Autodesk Inventor part; units mm, degrees
ref_plane "YZ Plane" through (0, 0, 0) normal (1, 0, 0) x (0, 1, 0)
ref_plane "XZ Plane" through (0, 0, 0) normal (0, 1, 0) x (-1, 0, 0)
ref_plane "XY Plane" through (0, 0, 0) normal (0, 0, 1) x (1, 0, 0)
sketch "Sketch1" plane through (0, 0, 0) normal (0, 1, 0) x (-1, 0, 0)
  line L0 (-62, 109.5) -> (62, 109.5)
  line L1 (62, 109.5) -> (62, -109.5)
  line L2 (62, -109.5) -> (-62, -109.5)
  line L3 (-62, -109.5) -> (-62, 109.5)
  line L4 (-62, 109.5) -> (62, -109.5) construction
  line L5 (62, 109.5) -> (-62, -109.5) construction
  point P0 (0, 0)
  dimension "d0" = 219
  dimension "d1" = 124
extrude "Extrusion1" add sketch "Sketch1" along normal blind 0.1
chamfer "Chamfer1" distance 4 angle 45 1 edges at (-62, 0.05, 109.5)
sketch "Sketch2" plane through (0, 0.1, 0) normal (0, 1, 0) x (1, 0, 0)
  line L0 (-35.5, -100.5) -> (-35.5, -70.5)
  line L1 (-35.5, -70.5) -> (-57.5, -70.5)
  line L2 (-62, 109.5) -> (-62, -109.5)
  line L3 (-62, -109.5) -> (62, -109.5)
  arc A0 (-57.5, -99) -> (-56, -100.5) centre (-57.5, -100.5) ccw
  line L4 (-35.5, -100.5) -> (-56, -100.5)
  line L5 (-57.5, -99) -> (-57.5, -70.5)
  line L6 (62, -109.5) -> (62, 109.5)
  line L7 (-35.5, -43.5) -> (-35.5, -13.5)
  line L8 (-35.5, -43.5) -> (-56, -43.5)
  line L9 (-35.5, -13.5) -> (-57.5, -13.5)
  line L10 (-57.5, -42) -> (-57.5, -13.5)
  arc A1 (-57.5, -42) -> (-56, -43.5) centre (-57.5, -43.5) ccw
  line L11 (-35.5, 13.5) -> (-35.5, 43.5)
  line L12 (-35.5, 13.5) -> (-56, 13.5)
  line L13 (-35.5, 43.5) -> (-57.5, 43.5)
  line L14 (-57.5, 15) -> (-57.5, 43.5)
  arc A2 (-57.5, 15) -> (-56, 13.5) centre (-57.5, 13.5) ccw
  line L15 (-35.5, 70.5) -> (-35.5, 100.5)
  line L16 (-35.5, 70.5) -> (-56, 70.5)
  line L17 (-35.5, 100.5) -> (-57.5, 100.5)
  line L18 (-57.5, 72) -> (-57.5, 100.5)
  arc A3 (-57.5, 72) -> (-56, 70.5) centre (-57.5, 70.5) ccw
  line L19 (-4.5, -100.5) -> (-4.5, -70.5)
  line L20 (-4.5, -100.5) -> (-25, -100.5)
  line L21 (-4.5, -70.5) -> (-26.5, -70.5)
  line L22 (-26.5, -99) -> (-26.5, -70.5)
  arc A4 (-26.5, -99) -> (-25, -100.5) centre (-26.5, -100.5) ccw
  line L23 (-4.5, -43.5) -> (-4.5, -13.5)
  line L24 (-4.5, -43.5) -> (-25, -43.5)
  line L25 (-4.5, -13.5) -> (-26.5, -13.5)
  line L26 (-26.5, -42) -> (-26.5, -13.5)
  arc A5 (-26.5, -42) -> (-25, -43.5) centre (-26.5, -43.5) ccw
  line L27 (-4.5, 13.5) -> (-4.5, 43.5)
  line L28 (-4.5, 13.5) -> (-25, 13.5)
  line L29 (-4.5, 43.5) -> (-26.5, 43.5)
  line L30 (-26.5, 15) -> (-26.5, 43.5)
  arc A6 (-26.5, 15) -> (-25, 13.5) centre (-26.5, 13.5) ccw
  line L31 (-4.5, 70.5) -> (-4.5, 100.5)
  line L32 (-4.5, 70.5) -> (-25, 70.5)
  line L33 (-4.5, 100.5) -> (-26.5, 100.5)
  line L34 (-26.5, 72) -> (-26.5, 100.5)
  arc A7 (-26.5, 72) -> (-25, 70.5) centre (-26.5, 70.5) ccw
  line L35 (26.5, -100.5) -> (26.5, -70.5)
  line L36 (26.5, -100.5) -> (6, -100.5)
  line L37 (26.5, -70.5) -> (4.5, -70.5)
  line L38 (4.5, -99) -> (4.5, -70.5)
  arc A8 (4.5, -99) -> (6, -100.5) centre (4.5, -100.5) ccw
  line L39 (26.5, -43.5) -> (26.5, -13.5)
  line L40 (26.5, -43.5) -> (6, -43.5)
  line L41 (26.5, -13.5) -> (4.5, -13.5)
  line L42 (4.5, -42) -> (4.5, -13.5)
  arc A9 (4.5, -42) -> (6, -43.5) centre (4.5, -43.5) ccw
  line L43 (26.5, 13.5) -> (26.5, 43.5)
  line L44 (26.5, 13.5) -> (6, 13.5)
  line L45 (26.5, 43.5) -> (4.5, 43.5)
  line L46 (4.5, 15) -> (4.5, 43.5)
  arc A10 (4.5, 15) -> (6, 13.5) centre (4.5, 13.5) ccw
  line L47 (26.5, 70.5) -> (26.5, 100.5)
  line L48 (26.5, 70.5) -> (6, 70.5)
  line L49 (26.5, 100.5) -> (4.5, 100.5)
  line L50 (4.5, 72) -> (4.5, 100.5)
  arc A11 (4.5, 72) -> (6, 70.5) centre (4.5, 70.5) ccw
  line L51 (57.5, -100.5) -> (57.5, -70.5)
  line L52 (57.5, -100.5) -> (37, -100.5)
  line L53 (57.5, -70.5) -> (35.5, -70.5)
  line L54 (35.5, -99) -> (35.5, -70.5)
  arc A12 (35.5, -99) -> (37, -100.5) centre (35.5, -100.5) ccw
  line L55 (57.5, -43.5) -> (57.5, -13.5)
  line L56 (57.5, -43.5) -> (37, -43.5)
  line L57 (57.5, -13.5) -> (35.5, -13.5)
  line L58 (35.5, -42) -> (35.5, -13.5)
  arc A13 (35.5, -42) -> (37, -43.5) centre (35.5, -43.5) ccw
  line L59 (57.5, 13.5) -> (57.5, 43.5)
  line L60 (57.5, 13.5) -> (37, 13.5)
  line L61 (57.5, 43.5) -> (35.5, 43.5)
  line L62 (35.5, 15) -> (35.5, 43.5)
  arc A14 (35.5, 15) -> (37, 13.5) centre (35.5, 13.5) ccw
  line L63 (57.5, 70.5) -> (57.5, 100.5)
  line L64 (57.5, 70.5) -> (37, 70.5)
  line L65 (57.5, 100.5) -> (35.5, 100.5)
  line L66 (35.5, 72) -> (35.5, 100.5)
  arc A15 (35.5, 72) -> (37, 70.5) centre (35.5, 70.5) ccw
  dimension "d46" = 1.5
  dimension "d47" = 30
  dimension "d50" = 9
  dimension "d51" = 4.5
  dimension "d62" = 57
  dimension "d65" = 31
  dimension "d77" = 22
extrude "Extrusion2" cut sketch "Sketch2" against normal through all
fillet "Fillet1" radius 1 5 edges at (62, 0.05, 109.5) (-58, 0.05, 109.5) (-62, 0.05, 105.5) (62, 0.05, -109.5) (-62, 0.05, -109.5)
sketch "Sketch3" plane through (0, 0.1, 0) normal (0, 1, 0) x (1, 0, 0)
  line L0 (-62, 108.5) -> (-62, -105.0858)
  line L1 (62, -108.5) -> (62, 108.5)
  line L2 (-57.5858, -109.5) -> (61, -109.5)
  line L3 (61, 109.5) -> (-61, 109.5)
  point P0 (0, 0)
  point P1 (-47, -105.5)
  point P2 (47, -105.5)
  point P3 (47, 105.5)
  point P4 (-47, 105.5)
  point P5 (-47, 0)
  point P6 (47, 0)
  dimension "d90" = 15
  dimension "d91" = 15
  dimension "d92" = 4
  dimension "d93" = 4
hole "Hole1" at (-47, 0.1, 105.5) at (47, 0.1, 105.5) at (47, 0.1, -105.5) at (-47, 0.1, -105.5) at (-47, 0.1, 0) at (47, 0.1, 0) direction (0, -1, 0) diameter 3.4 end through all
properties part number "Assembly Stencil" material "Stainless Steel"
CAD build for the part. Positions are in the model's coordinates, mm. Give positions to 0.01 mm unless a question says otherwise; leave off trailing zeros. Loops run counter-clockwise (first coordinate to the right, second up) from the corner with the lowest first, then second, coordinate; pieces in that order, holes last. Notation, with made-up numbers: (23.25, 33) -> (71.25, 33) arc R23 cw to (71.25, 57) -> close; hole circle Ø3 at (-20, -19.75). An arc over 180 degrees is marked (long way). Use a Markdown table: item, result.
1. Slice it at A-A (z = -26). List the corners of the cut face in (x, y), plus the area to 3 significant figures.
Check result:
| item | result |
|---|---|
| outline | (-62, 0) -> (-57.5, 0) -> (-57.5, 0.1) -> (-62, 0.1) -> close; (-35.5, 0) -> (-26.5, 0) -> (-26.5, 0.1) -> (-35.5, 0.1) -> close; (-4.5, 0) -> (4.5, 0) -> (4.5, 0.1) -> (-4.5, 0.1) -> close; (26.5, 0) -> (35.5, 0) -> (35.5, 0.1) -> (26.5, 0.1) -> close; (57.5, 0) -> (62, 0) -> (62, 0.1) -> (57.5, 0.1) -> close |
| area | 3.60 mm^2 |
2. Slice it at B-B (x = -21). List the corners of the cut face in (y, z), plus the area to 3 significant figures.
Check result:
| item | result |
|---|---|
| outline | (0, -109.5) -> (0.1, -109.5) -> (0.1, -100.5) -> (0, -100.5) -> close; (0, -70.5) -> (0.1, -70.5) -> (0.1, -43.5) -> (0, -43.5) -> close; (0, -13.5) -> (0.1, -13.5) -> (0.1, 13.5) -> (0, 13.5) -> close; (0, 43.5) -> (0.1, 43.5) -> (0.1, 70.5) -> (0, 70.5) -> close; (0, 100.5) -> (0.1, 100.5) -> (0.1, 109.5) -> (0, 109.5) -> close |
| area | 9.90 mm^2 |
3. Wall check: L1, parallel to Z at x = -24, y = 0.05; L2, parallel to X at y = 0.05, z = 105.5. Give the ranges that are in metal, low to high. Write a range as [from, to].
Check result:
| item | result |
|---|---|
| L1 | z = [-109.5, -100.5], [-70.5, -43.5], [-13.5, 13.5], [43.5, 70.5], [100.5, 109.5] |
| L2 | x = [-61.91, -48.7], [-45.3, 45.3], [48.7, 62] |
